Source: three-view drawing plus pictorial views. Frame: mm from the lowest corner of the part. Give positions to 0.01 mm unless a question says otherwise; leave off trailing zeros. Order: outer loops, then holes, each group sorted by start corner. A loop starts at its lowest first (then second) coordinate and runs counter-clockwise, first axis right, second up.
1) Section B-B, the plane x = 12. Return loops of the section in (y, z), plus the area to 3 significant figures.
2) Section C-C, the plane z = 2. Return loops of the section in (x, y), plus the area to 3 significant figures.
3) Material intervals for line 1 (Y direction, x = 20, z = 5.25); line 2 (X direction, y = 21.5, z = 5.5); line 3 (X direction, y = 4, z = 1.5), sorted ascending.
4) Section A-A, the plane y = 19.5. Return loops of the section in (x, z), plus the area to 3 significant figures.
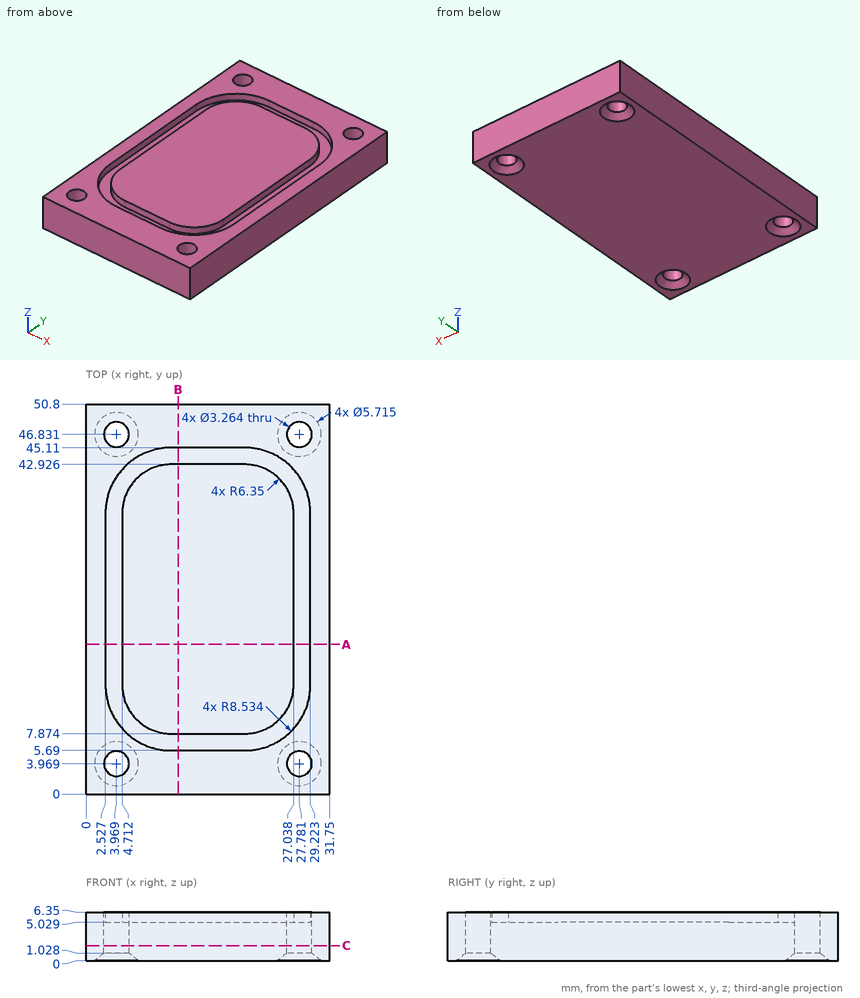
From the geometry:
1. outline: (0, 0) - (50.8, 0) - (50.8, 6.35) - (45.11, 6.35) - (45.11, 5.03) - (42.93, 5.03) - (42.93, 6.35) - (7.87, 6.35) - (7.87, 5.03) - (5.69, 5.03) - (5.69, 6.35) - (0, 6.35) - close
1. area: 317 mm2
2. outline: (0, 0) - (31.75, 0) - (31.75, 50.8) - (0, 50.8) - close; hole circle Ø3.26 at (3.97, 3.97); hole circle Ø3.26 at (3.97, 46.83); hole circle Ø3.26 at (27.78, 3.97); hole circle Ø3.26 at (27.78, 46.83)
2. area: 1,580 mm2
3. line 1: y = 0 to 5.69, 7.87 to 42.93, 45.11 to 50.8
3. line 2: x = 0 to 2.53, 4.71 to 27.04, 29.22 to 31.75
3. line 3: x = 0 to 2.34, 5.6 to 26.15, 29.41 to 31.75
4. outline: (0, 0) - (31.75, 0) - (31.75, 6.35) - (29.22, 6.35) - (29.22, 5.03) - (27.04, 5.03) - (27.04, 6.35) - (4.71, 6.35) - (4.71, 5.03) - (2.53, 5.03) - (2.53, 6.35) - (0, 6.35) - close
4. area: 196 mm2
